from build123d import *

# Parameters (mm, degrees)
SKETCH_W        = 62
SKETCH_H        = 83.956
PAD_DEPTH       = 1.6
SKETCH001_W     = 62
SKETCH001_H     = 83.956
SKETCH001_W_2   = 58
SKETCH001_H_2   = 79.956
PAD001_DEPTH    = 17.6
PAD002_DEPTH    = 41.978
SKETCH003_R     = 4
SKETCH003_R_2   = 2
SKETCH003_R_3   = 2.5
SKETCH003_R_4   = 1.15
PAD003_DEPTH    = 6.1
PAD004_START    = -10
PAD004_DEPTH    = 5
SKETCH005_W     = 21.5
SKETCH005_H     = 1.5
SKETCH005_H_2   = 2.022
SKETCH005_W_2   = 58
PAD005_DEPTH    = 8.066667
SKETCH010_W     = 58
SKETCH010_H     = 35.956
POCKET006_DEPTH = 17.6
PAD008_DEPTH    = 11.2
SKETCH012_W     = 16
SKETCH012_H     = 8
POCKET003_DEPTH = 16
SKETCH013_R     = 2
POCKET004_DEPTH = 8


with BuildPart() as part:
    # Sketch → Pad (new body)
    with BuildSketch(Plane.XY):
        Rectangle(SKETCH_W, SKETCH_H)
        with BuildLine():
            ThreePointArc((7.5, 7.5), (0, 15), (-7.5, 7.5))
            Line((-7.5, 7.5), (-7.5, -7.5))
            ThreePointArc((-7.5, -7.5), (0, -15), (7.5, -7.5))
            Line((7.5, -7.5), (7.5, 7.5))
        make_face(mode=Mode.SUBTRACT)
    extrude(amount=PAD_DEPTH)

    # Sketch001 → Pad001 (join)
    with BuildSketch(Plane.XY):
        Rectangle(SKETCH001_W, SKETCH001_H)
        Rectangle(SKETCH001_W_2, SKETCH001_H_2, mode=Mode.SUBTRACT)
    extrude(amount=PAD001_DEPTH)

    # Sketch002 → Pad002 (join, symmetric)
    with BuildSketch(Plane.XZ):
        Polygon((-29, 17.6), (-29, 2.257725), (-22, 10.6), (-22, 17.6), align=None)
        Polygon((22, 17.6), (22, 10.6), (29, 2.257725), (29, 17.6), align=None)
    extrude(amount=PAD002_DEPTH, both=True)

    # Sketch003 → Pad003 (join)
    with BuildSketch(Plane.XY):
        with Locations((16, 34.478)):
            Circle(SKETCH003_R)
        with Locations((16, 34.478)):
            Circle(SKETCH003_R_2, mode=Mode.SUBTRACT)
        with Locations((16, 12.478)):
            Circle(SKETCH003_R)
        with Locations((16, 12.478)):
            Circle(SKETCH003_R_2, mode=Mode.SUBTRACT)
        with Locations((-15, 23.478)):
            Circle(SKETCH003_R_3)
        with Locations((-15, 23.478)):
            Circle(SKETCH003_R_4, mode=Mode.SUBTRACT)
    extrude(amount=PAD003_DEPTH)

    # Sketch004 → Pad004 (join)
    with BuildSketch(Plane.YZ.offset(PAD004_START)):
        Polygon((-30.978, 0), (-30.978, 4.1), (-39.978, 4.1), (-39.978, 3.1), (-31.978, 3.1), (-31.978, 0), align=None)
    extrude(amount=-PAD004_DEPTH)

    # Sketch005 → Pad005 (join)
    with BuildSketch(Plane.XY.offset(1.6)):
        with Locations((18.25, 6.228)):
            Rectangle(SKETCH005_W, SKETCH005_H)
        with Locations((-18.25, 6.489)):
            Rectangle(SKETCH005_W, SKETCH005_H_2)
        with Locations((0, -31.228)):
            Rectangle(SKETCH005_W_2, SKETCH005_H)
    extrude(amount=PAD005_DEPTH)

    # Sketch010 → Pocket006 (cut)
    with BuildSketch(Plane.XY.offset(1.6)):
        with Locations((0, -12.5)):
            Rectangle(SKETCH010_W, SKETCH010_H)
    extrude(amount=POCKET006_DEPTH, mode=Mode.SUBTRACT)

    # Sketch011 → Pad008 (join)
    with BuildSketch(Plane.XY):
        with BuildLine():
            Line((-10.3, 41.978), (10.3, 41.978))
            ThreePointArc((8.8, 43.478), (9.23934, 42.41734), (10.3, 41.978))
            Line((8.8, 56.078), (8.8, 43.478))
            ThreePointArc((8.8, 56.078), (8.36066, 57.13866), (7.3, 57.578))
            Line((-7.3, 57.578), (7.3, 57.578))
            ThreePointArc((-7.3, 57.578), (-8.36066, 57.13866), (-8.8, 56.078))
            Line((-8.8, 56.078), (-8.8, 43.478))
            ThreePointArc((-10.3, 41.978), (-9.23934, 42.41734), (-8.8, 43.478))
        make_face()
    extrude(amount=PAD008_DEPTH)

    # Sketch012 → Pocket003 (cut)
    with BuildSketch(Plane(origin=(0, 39.978, 0), x_dir=(-1, 0, 0), z_dir=(0, 1, 0))):
        with Locations((0, 5.6)):
            Rectangle(SKETCH012_W, SKETCH012_H)
    extrude(amount=POCKET003_DEPTH, mode=Mode.SUBTRACT)

    # Sketch013 (on DatumPlane) → Pocket004 (cut)
    with BuildSketch(Plane.XY.offset(17.6)):
        with Locations((-26.5, 37.478)):
            Circle(SKETCH013_R)
        with Locations((-26.5, -37.478)):
            Circle(SKETCH013_R)
        with Locations((26.5, -37.478)):
            Circle(SKETCH013_R)
        with Locations((26.5, 37.478)):
            Circle(SKETCH013_R)
        with Locations((-26.5, 20.522)):
            Circle(SKETCH013_R)
        with Locations((26.5, 20.522)):
            Circle(SKETCH013_R)
    extrude(amount=-POCKET004_DEPTH, mode=Mode.SUBTRACT)


with BuildPart() as part_1:
    # Body placement: moved
    add(part.part.moved(Location((0, 0, -45))))


solid = part_1.part
Here's how the part is built. I have some questions about the finished solid (model axes, mm). A direction names the side the tool comes from. Round coordinates to 2 decimals unless told otherwise and drop trailing zeros. Order: outer loops, then holes, each group sorted by start corner. A loop starts at its lowest first (then second) coordinate and runs counter-clockwise, first axis right, second up. Notation, with made-up numbers: (-38, 9.25) -> (10, 9.25) arc R23 cw to (10, 41.25) -> close; hole circle Ø7 at (58, 85). An arc over 180 degrees is marked (long way). Return JSON: item names as keys, results as strings.
Q1. If we section it at D-D on x = 26.5: List the corners of the cut face in (y, z) for me, plus the area to 3 significant figures.
Filled sheet:
{"outline": "(-41.98, -45) -> (41.98, -45) -> (41.98, -27.4) -> (39.48, -27.4) -> (39.48, -35.4) -> (35.48, -35.4) -> (35.48, -27.4) -> (22.52, -27.4) -> (22.52, -35.4) -> (18.52, -35.4) -> (18.52, -27.4) -> (5.48, -27.4) -> (5.48, -43.4) -> (-30.48, -43.4) -> (-30.48, -27.4) -> (-35.48, -27.4) -> (-35.48, -35.4) -> (-39.48, -35.4) -> (-39.48, -27.4) -> (-41.98, -27.4) -> close; hole (-39.98, -43.4) -> (-31.98, -43.4) -> (-31.98, -39.76) -> (-39.98, -39.76) -> close; hole (6.98, -43.4) -> (39.98, -43.4) -> (39.98, -39.76) -> (6.98, -39.76) -> close", "area": "657 mm^2"}
Q2. If we section it at A-A on y = 0: List the corners of the cut face in (x, z) for me, plus the area to 3 significant figures.
Filled sheet:
{"outline": "(-31, -45) -> (-7.5, -45) -> (-7.5, -43.4) -> (-29, -43.4) -> (-29, -27.4) -> (-31, -27.4) -> close; (7.5, -45) -> (31, -45) -> (31, -27.4) -> (29, -27.4) -> (29, -43.4) -> (7.5, -43.4) -> close", "area": "139 mm^2"}
Q3. Which directions (+Z, -Z, +X, -X, +Y, -Y) give clear straight access to the entire face, cutting with the end or side of a thin tool? Please do faces 1 (the cylindrical face through (0, 15, -44)), 2 (the flat face through (-8, 48, -39)), 3 (the flat face through (22, -35, -31)).
Filled sheet:
{"face 1": "+Z, -Z", "face 2": "none", "face 3": "+Z"}
Q4. I need wall thicknesses on line 1 along Y through (x, z) = (-17, -35.5); line 2 along Y through (x, z) = (12.5, -36.75); line 3 along Y through (x, z) = (26.5, -33). Which ranges of each line are inside material? Lowest first, please. Write a range as from..to.
Filled sheet:
{"line 1": "y = -41.98..-39.98, -31.98..-30.48, 5.48..7.5, 39.98..41.98", "line 2": "y = -41.98..-39.98, -31.98..-30.48, 5.48..6.98, 39.98..41.98", "line 3": "y = -41.98..-39.48, -35.48..-30.48, 5.48..18.52, 22.52..35.48, 39.48..41.98"}
Q5. For pin 1 Ø8 at (x, y) = (-1.5, 50.5) entering from +Z; pin 2 Ø6.5 at (x, z) = (-19.5, -39) entering from +Y; pin 3 Ø5 at (x, y) = (16, 34.478) entering from +Z, each with a flat end and sliding along its axis, tell me the tip position at first contact or that it passes through.
Filled sheet:
{"pin 1": "stops at z = -33.8", "pin 2": "stops at y = 41.98", "pin 3": "stops at z = -38.9"}
Q6. If we section it at B-B on y = 49.5: List the corners of the cut face in (x, z) for me.
Filled sheet:
{"outline": "(-8.8, -45) -> (8.8, -45) -> (8.8, -33.8) -> (-8.8, -33.8) -> close; hole (-8, -43.4) -> (8, -43.4) -> (8, -35.4) -> (-8, -35.4) -> close"}
Q7. If we mould it in two halves opening along X, with no side actions, what happens to faces 4 (the flat face through (31, -1, -36)), 5 (the flat face through (-23, 13, -27.4)), 6 (the flat face through (8, 48, -39))? For each: released by +X, released by -X, zero draft, split by the parting line, or undercut.
Filled sheet:
{"face 4": "released by +X", "face 5": "zero draft", "face 6": "undercut"}
Q8. If we section it at C-C on x = 0: List the corners of the cut face in (y, z) for me.
Filled sheet:
{"outline": "(-41.98, -45) -> (-15, -45) -> (-15, -43.4) -> (-30.48, -43.4) -> (-30.48, -35.33) -> (-31.98, -35.33) -> (-31.98, -43.4) -> (-39.98, -43.4) -> (-39.98, -27.4) -> (-41.98, -27.4) -> close; (15, -45) -> (57.58, -45) -> (57.58, -33.8) -> (41.98, -33.8) -> (41.98, -27.4) -> (39.98, -27.4) -> (39.98, -35.4) -> (55.98, -35.4) -> (55.98, -43.4) -> (15, -43.4) -> close"}
